```python
from build123d import *

# Parameters (mm, degrees)
SKETCH1_R           = 3
SKETCH1_R_2         = 1.7
BOSS_EXTRUDE1_DEPTH = 3
BOSS_EXTRUDE2_START = -3
SKETCH1_3_R         = 4
SKETCH1_3_R_2       = 3
BOSS_EXTRUDE2_DEPTH = 3


with BuildPart() as part:
    # Sketch1 → Boss-Extrude1 (new body)
    with BuildSketch(Plane.XY):
        with BuildLine():
            ThreePointArc((-6, 2), (0, -4), (6, 2))
            Line((6, 2), (6, 4))
            ThreePointArc((6, 4), (0, 10), (-6, 4))
            Line((-6, 4), (-6, 2))
        make_face()
        Circle(SKETCH1_R, mode=Mode.SUBTRACT)
        with Locations((0, 7.5)):
            Circle(SKETCH1_R_2, mode=Mode.SUBTRACT)
    extrude(amount=BOSS_EXTRUDE1_DEPTH)

    # Sketch1_3 → Boss-Extrude2 (add)
    with BuildSketch(Plane.XY.offset(BOSS_EXTRUDE2_START)):
        Circle(SKETCH1_3_R)
        Circle(SKETCH1_3_R_2, mode=Mode.SUBTRACT)
    extrude(amount=BOSS_EXTRUDE2_DEPTH)


solid = part.part
```
Geometry: final body of the model. Coordinates: model frame, mm. A direction names the side the tool comes from. Round coordinates to 2 decimals unless told otherwise and drop trailing zeros. Order: outer loops, then holes, each group sorted by start corner. A loop starts at its lowest first (then second) coordinate and runs counter-clockwise, first axis right, second up. Notation, with made-up numbers: M 12.5,41.25 L 67.5,41.25 A19 ccw 67.5,50.25 Z; hole C 88,22.5 d3. An arc over 180 degrees is marked long. Use one line per item in the form item = value. Start each with the question number.
Q1. Access query for faces 4 (the face through (-3, 0, 0)), 5 (the face through (-0.867, -3.905, -1.521)). Directions: +Z, -Z, +X, -X, +Y, -Y. A direction counts if a zero-diameter tool reaches every point of the face in a straight line with its end or side. Return the directions, or none.
Q2. Cut plane B-B (x = -1). Return loops of the section in (y, z).
Q3. Pin query (flat end, axial travel): pin 1 Ø3 at (x, z) = (3, -1) entering from -Y; pin 2 Ø1.5 at (x, z) = (3, -0.5) entering from -Y; pin 3 Ø1 at (y, z) = (3, -2) entering from -X. Return the tip coordinate at first contact, or that it passes through.
Q4. Cut plane A-A (y = 1). Return loops of the section in (x, z), and give its area (3 significant figures).
Q5. Cut plane D-D (z = -1.5). Return loops of the section in (x, y), and give its area (3 significant figures).
Q6. Material intervals for line 1 (Y direction, x = 0, z = 2.25); line 2 (Y direction, x = 0, z = -1.05); line 3 (X direction, y = 1.25, z = -0.85), sorted ascending. Write a range as [from, to].
Q7. Mould query, pull axis Z, two halves, no side actions, for faces 1 (the face through (0, 5, 0)), 2 (the face through (0, 5, 3)), 3 (the face through (6, 3, 1)). Classes: +Z half, -Z half, draft (parallel to the pull), parting line (faces both ways), or undercut.
Q8. Cut plane C-C (z = 0.8). Return loops of the section in (x, y), and give its area (3 significant figures).
Geometry results:
q1.face_4 = +Z, -Z
q1.face_5 = -Z
q2.outline = M -3.92,0 L -3.87,0 L -3.87,-3 L -2.83,-3 L -2.83,3 L -3.92,3 Z; M 2.83,-3 L 3.87,-3 L 3.87,0 L 6.13,0 L 6.13,3 L 2.83,3 Z; M 8.87,0 L 9.92,0 L 9.92,3 L 8.87,3 Z
q3.pin_1 = -3.71
q3.pin_2 = -3.48
q3.pin_3 = -3.12
q4.outline = M -5.92,0 L -3.87,0 L -3.87,-3 L -2.83,-3 L -2.83,3 L -5.92,3 Z; M 2.83,-3 L 3.87,-3 L 3.87,0 L 5.92,0 L 5.92,3 L 2.83,3 Z
q4.area = 24.8 mm^2
q5.outline = C 0,0 d8; hole C 0,0 d6
q5.area = 22.0 mm^2
q6.line_1 = [-4, -3], [3, 5.8], [9.2, 10]
q6.line_2 = [-4, -3], [3, 4]
q6.line_3 = [-3.8, -2.73], [2.73, 3.8]
q7.face_1 = -Z half
q7.face_2 = +Z half
q7.face_3 = draft
q8.outline = M -6,2 A6 ccw 6,2 L 6,4 A6 ccw -6,4 Z; hole C 0,0 d6; hole C 0,7.5 d3.4
q8.area = 99.7 mm^2
